```python
from build123d import *

# Parameters (mm, degrees)
SKETCH1_W           = 20
SKETCH1_H           = 25
BOSS_EXTRUDE1_DEPTH = 170
SHELL1_T            = -1
SKETCH2_R           = 3.5
CUT_EXTRUDE1_DEPTH  = 170


with BuildPart() as part:
    # Sketch1 → Boss-Extrude1 (new body)
    with BuildSketch(Plane.XY):
        with Locations((-15.769295372, -6.071428571)):
            Rectangle(SKETCH1_W, SKETCH1_H)
    extrude(amount=BOSS_EXTRUDE1_DEPTH)

    # Shell1
    shell1_openings = [part.faces().sort_by_distance(p)[0] for p in [
        (-15.769295372, -6.071428571, 170),
        (-15.769295372, -6.071428571, 0),
    ]]
    offset(amount=SHELL1_T, openings=shell1_openings, kind=Kind.INTERSECTION)

    # Sketch2 → Cut-Extrude1 (cut)
    with BuildSketch(Plane.ZY.offset(25.769295372)):
        with Locations(Location((15, -6.071428571, 0), (0, 0, 270))):
            Circle(SKETCH2_R)
        with Locations(Location((155, -6.071428571, 0), (0, 0, 270))):
            Circle(SKETCH2_R)
    extrude(amount=-CUT_EXTRUDE1_DEPTH, mode=Mode.SUBTRACT)


solid = part.part
```
Build history of the part. All positions in model axes, mm. A direction names the side the tool comes from. Give positions to 0.01 mm unless a question says otherwise; leave off trailing zeros. Order: outer loops, then holes, each group sorted by start corner. A loop starts at its lowest first (then second) coordinate and runs counter-clockwise, first axis right, second up. Notation, with made-up numbers: M 52,7 L 85,7 A18 cw 85,24 Z; hole C 1.5,-5 d4. An arc over 180 degrees is marked long. Write item = value, one per line. Start each with the question number.
(1) Which spindle directions (+Z, -Z, +X, -X, +Y, -Y) get a long thin tool onto all of the face, cutting with end or side? Do faces 4 (the flat face through (-6.769, -6, 84)), 5 (the cylindrical face through (-6.276, -5.313, 11.583)). Say none if no direction does.
(2) Slice it at B-B on y = -15. Write the cut outline in (x, z).
(3) Slice it at A-A on x = -11.5. Write the cut outline in (y, z).
(4) Slice it at C-C on z = 155. Write the cut outline in (x, y).
(5) Slice it at D-D on z = 123. Write the cut outline in (x, y).
(6) Two-plate mould, pull along Z, no slides. Class faces 1 (the cylindrical face through (-6.276, -5.313, 151.583)), 2 (the flat face through (-24.769, -6, 84)), 3 (the flat face through (-25, -6, 170)): released by +Z, released by -Z, zero draft, split by the parting line, or undercut.
(7) Probe L1, parallel to X at y = -12, z = 49; L2, parallel to Y at x = -15, z = 58; L3, parallel to Y at x = -6.05, z = 155. List the from-to ranges inside material, lowest first. Write a range as [from, to].
Responses:
q1.face_4 = +Z, -Z
q1.face_5 = +X, -X
q2.outline = M -25.77,0 L -24.77,0 L -24.77,170 L -25.77,170 Z; M -6.77,0 L -5.77,0 L -5.77,170 L -6.77,170 Z
q3.outline = M -18.57,0 L -17.57,0 L -17.57,170 L -18.57,170 Z; M 5.43,0 L 6.43,0 L 6.43,170 L 5.43,170 Z
q4.outline = M -25.77,-18.57 L -5.77,-18.57 L -5.77,-9.57 L -6.77,-9.57 L -6.77,-17.57 L -24.77,-17.57 L -24.77,-9.57 L -25.77,-9.57 Z; M -25.77,-2.57 L -24.77,-2.57 L -24.77,5.43 L -6.77,5.43 L -6.77,-2.57 L -5.77,-2.57 L -5.77,6.43 L -25.77,6.43 Z
q5.outline = M -25.77,-18.57 L -5.77,-18.57 L -5.77,6.43 L -25.77,6.43 Z; hole M -24.77,-17.57 L -6.77,-17.57 L -6.77,5.43 L -24.77,5.43 Z
q6.face_1 = undercut
q6.face_2 = zero draft
q6.face_3 = released by +Z
q7.L1 = [-25.77, -24.77], [-6.77, -5.77]
q7.L2 = [-18.57, -17.57], [5.43, 6.43]
q7.L3 = [-18.57, -9.57], [-2.57, 6.43]
